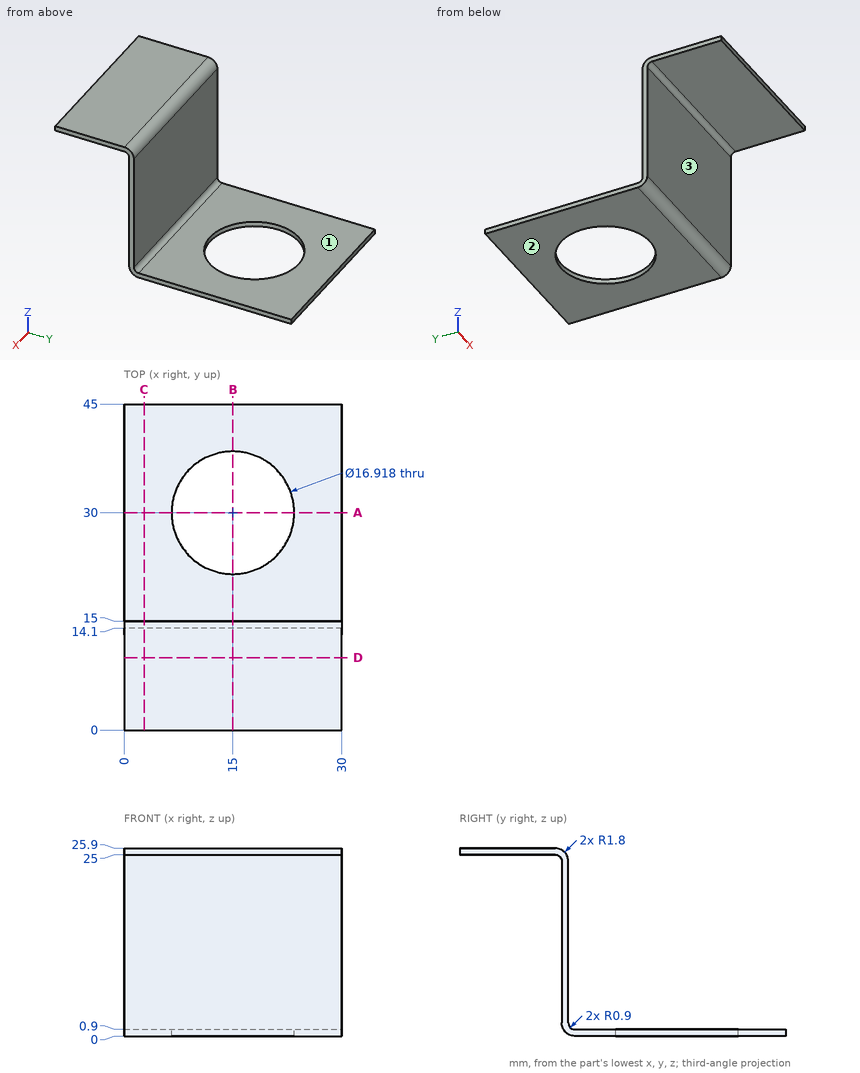
Here's the drawing with two shaded views (mm, measured from the low corner). I have some questions. A direction names the side the tool comes from. Round coordinates to 2 decimals unless told otherwise and drop trailing zeros. Write each loop counter-clockwise with the first axis right and the second up, starting at its lowest first coordinate (ties: lowest second). Pieces come first, ordered by that corner, then holes.
(1) Suppose I cut it at C-C on x = 2.75. Write out the boundary of the cut face in (y, z).
Findings below:
outline: (0, 25) - (13.2, 25) arc R0.9 cw to (14.1, 24.1) - (14.1, 1.8) arc R1.8 ccw to (15.9, 0) - (45, 0) - (45, 0.9) - (15.9, 0.9) arc R0.9 cw to (15, 1.8) - (15, 24.1) arc R1.8 ccw to (13.2, 25.9) - (0, 25.9) - close
(2) If I drill on probe 1 along X at (y, z) = (30, 0.65); probe 2 along Z at (x, y) = (23.25, 23); probe 3 along Z at (x, y) = (13.25, 10), over which ranges is the centre line in solid material (lowest first)?
Findings below:
probe 1: x = 0 to 6.54, 23.46 to 30
probe 2: z = 0 to 0.9
probe 3: z = 25 to 25.9
(3) For pin 1 (11 mm diameter, centred on x = 17, z = 16.5, fed in from -Y); pin 2 (1.5 mm diameter, centred on x = 6.5, z = 5, fed in from +Y); pin 3 (1.5 mm diameter, centred on x = 24.5, y = 23, fed in from +Z), each with a flat end and sliding along its axis, tell me the tip position at first contact or that it passes through.
Findings below:
pin 1: stops at y = 14.1
pin 2: stops at y = 15
pin 3: stops at z = 0.9
(4) Suppose I cut it at B-B on x = 15. Write out the boundary of the cut face in (y, z).
Findings below:
outline: (0, 25) - (13.2, 25) arc R0.9 cw to (14.1, 24.1) - (14.1, 1.8) arc R1.8 ccw to (15.9, 0) - (21.54, 0) - (21.54, 0.9) - (15.9, 0.9) arc R0.9 cw to (15, 1.8) - (15, 24.1) arc R1.8 ccw to (13.2, 25.9) - (0, 25.9) - close; (38.46, 0) - (45, 0) - (45, 0.9) - (38.46, 0.9) - close
(5) Which directions (+Z, -Z, +X, -X, +Y, -Y) give clear straight access to the entire face, cutting with the end or side of a thin tool? Please do the marked faces 1, 2 and 3.
Findings below:
face 1: +Z, +X, -X, +Y
face 2: -Z, +X, -X, +Y, -Y
face 3: -Z, +X, -X, -Y
(6) Suppose I cut it at D-D on y = 10. Write out the boundary of the cut face in (x, z).
Findings below:
outline: (0, 25) - (30, 25) - (30, 25.9) - (0, 25.9) - close
(7) Suppose I cut it at A-A on y = 30. Write out the boundary of the cut face in (x, z).
Findings below:
outline: (0, 0) - (6.54, 0) - (6.54, 0.9) - (0, 0.9) - close; (23.46, 0) - (30, 0) - (30, 0.9) - (23.46, 0.9) - close
